Could you check a few things on this model? Use its own coordinates, in mm. Face numbers are marked on the shaded views. A direction names the side the tool comes from. Coordinates: 2 decimals unless noted, no trailing zeros. Order: outer loops, then holes, each group sorted by start corner. A loop starts at its lowest first (then second) coordinate and runs counter-clockwise, first axis right, second up. Notation, with made-up numbers: (-7.75, 65.5) -> (45.25, 65.5) arc R8 cw to (45.25, 78.5) -> close; hole circle Ø2 at (-24, 87.5). An arc over 180 degrees is marked (long way). Use a Markdown table: item, result. Add a question column.
1) If we section it at C-C (y = 3): Write out the boundary of the cut face in (x, z) (3 decimals).
2) Will these pins go through, and if not, where does the flat tip stop? pin 1 Ø1.9 at (y, z) = (1, 0) entering from +X; pin 2 Ø1.1 at (y, z) = (1.5, -0.5) entering from -X; pin 3 Ø1 at (y, z) = (6.5, 1) entering from +X.
3) Thinking about a two-plate mould opening in X: for the marked faces 1, 2 and 3, which applies, +X half, -X half, draft (parallel to the pull), parting line (faces both ways), or undercut?
4) If we section it at B-B (x = 0): Write out the boundary of the cut face in (y, z) (3 decimals), plus the area to 3 significant figures.
5) If we section it at D-D (y = 20.25): Write out the boundary of the cut face in (x, z).
6) Which directions (+Z, -Z, +X, -X, +Y, -Y) give clear straight access to the entire face, cutting with the end or side of a thin tool? Please do the marked faces 4, 5, 6, 7 and 8.
7) If we section it at A-A (z = 0): Write out the boundary of the cut face in (x, y), plus the area to 3 significant figures.
8) If I drill on L1, parallel to X at y = 13.75, z = 0; L2, parallel to X at y = 5.75, z = 0; L3, parallel to Z at x = 0.75, y = 24.25, over which ranges is the centre line in solid material (lowest first)? Write a range as [from, to].
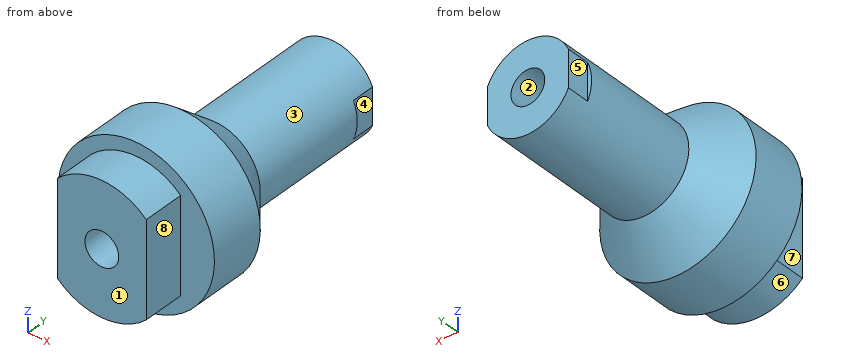
```python
from build123d import *

# Parameters (mm, degrees)
CORTE_EXTRUS_O1_DEPTH      = 27.95579715
CORTE_EXTRUS_O1_DEPTH_BACK = 27.95579715
ESBO_O2_W                  = 1.825
ESBO_O2_H                  = 3.75
ESBO_O2_W_2                = 0.35
ESBO_O2_H_2                = 2.1
CORTE_EXTRUS_O2_DEPTH      = 27.95579715
CORTE_EXTRUS_O2_DEPTH_BACK = 27.95579715
ESBO_O3_R                  = 1.5


with BuildPart() as part:
    # Esboço1 → Revolução1 (revolve)
    with BuildSketch(Plane.XY, mode=Mode.PRIVATE) as revolu_o1_sk:
        Polygon((-5.775, 0), (-5.775, 3.75), (-6.95, 3.75), (-6.95, 8.75), (-3.95, 12.4), (-3.95, 25.1), (0, 25.1), (0, 0), align=None)
    revolve(revolu_o1_sk.sketch.rotate(Axis((0, 0, 0), (0, 1, 0)), 270), axis=Axis((0, 0, 0), (0, 1, 0)))

    # Esboço2 → Corte-extrusão1 (cut, two sides: drawn at the far end of the back side and taken through both)
    with BuildSketch(Plane.XY.offset(-CORTE_EXTRUS_O1_DEPTH_BACK)):
        with Locations((-4.8625, 1.875)):
            Rectangle(ESBO_O2_W, ESBO_O2_H)
        with Locations((-3.775, 24.05)):
            Rectangle(ESBO_O2_W_2, ESBO_O2_H_2)
        with Locations((3.775, 24.05)):
            Rectangle(ESBO_O2_W_2, ESBO_O2_H_2)
        with Locations((4.8625, 1.875)):
            Rectangle(ESBO_O2_W, ESBO_O2_H)
    extrude(amount=CORTE_EXTRUS_O1_DEPTH + CORTE_EXTRUS_O1_DEPTH_BACK, mode=Mode.SUBTRACT)

    # Esboço3 → Corte-extrusão2 (cut, two sides: drawn at the far end of the back side and taken through both)
    with BuildSketch(Plane(origin=(0, 0, 0), x_dir=(1, 0, 0), z_dir=(0, 1, 0)).offset(-CORTE_EXTRUS_O2_DEPTH_BACK)):
        with Locations(Location((0, 0, 0), (0, 0, 270))):
            Circle(ESBO_O3_R)
    extrude(amount=CORTE_EXTRUS_O2_DEPTH + CORTE_EXTRUS_O2_DEPTH_BACK, mode=Mode.SUBTRACT)


solid = part.part
```
Answer sheet:
| question | item | result |
|---|---|---|
| 1 | outline | (-3.95, -4.213) arc R5.775 ccw to (3.95, -4.213) -> (3.95, 4.213) arc R5.775 ccw to (-3.95, 4.213) -> close; hole circle Ø3 at (0, 0) |
| 2 | pin 1 | x = 3.95 |
| 2 | pin 2 | x = -3.95 |
| 2 | pin 3 | x = 6.93 |
| 3 | face 1 | draft |
| 3 | face 2 | undercut |
| 3 | face 3 | parting line |
| 4 | outline | (0, -5.775) -> (3.75, -5.775) -> (3.75, -6.95) -> (8.75, -6.95) -> (12.4, -3.95) -> (25.1, -3.95) -> (25.1, -1.5) -> (0, -1.5) -> close; (0, 1.5) -> (25.1, 1.5) -> (25.1, 3.95) -> (12.4, 3.95) -> (8.75, 6.95) -> (3.75, 6.95) -> (3.75, 5.775) -> (0, 5.775) -> close |
| 4 | area | 178 mm2 |
| 5 | outline | circle Ø7.9 at (0, 0); hole circle Ø3 at (0, 0) |
| 6 | face 4 | +Z, -Z, +X, +Y |
| 6 | face 5 | +Z, -Z, -X, +Y |
| 6 | face 6 | -Z, -Y |
| 6 | face 7 | +Z, -Z, -X, -Y |
| 6 | face 8 | +Z, -Z, +X, -Y |
| 7 | outline | (-6.95, 3.75) -> (-3.95, 3.75) -> (-3.95, 0) -> (-1.5, 0) -> (-1.5, 25.1) -> (-3.6, 25.1) -> (-3.6, 23) -> (-3.95, 23) -> (-3.95, 12.4) -> (-6.95, 8.75) -> close; (1.5, 0) -> (3.95, 0) -> (3.95, 3.75) -> (6.95, 3.75) -> (6.95, 8.75) -> (3.95, 12.4) -> (3.95, 23) -> (3.6, 23) -> (3.6, 25.1) -> (1.5, 25.1) -> close |
| 7 | area | 162 mm2 |
| 8 | L1 | [-3.95, -1.5], [1.5, 3.95] |
| 8 | L2 | [-6.95, -1.5], [1.5, 6.95] |
| 8 | L3 | [-3.88, -1.3], [1.3, 3.88] |
